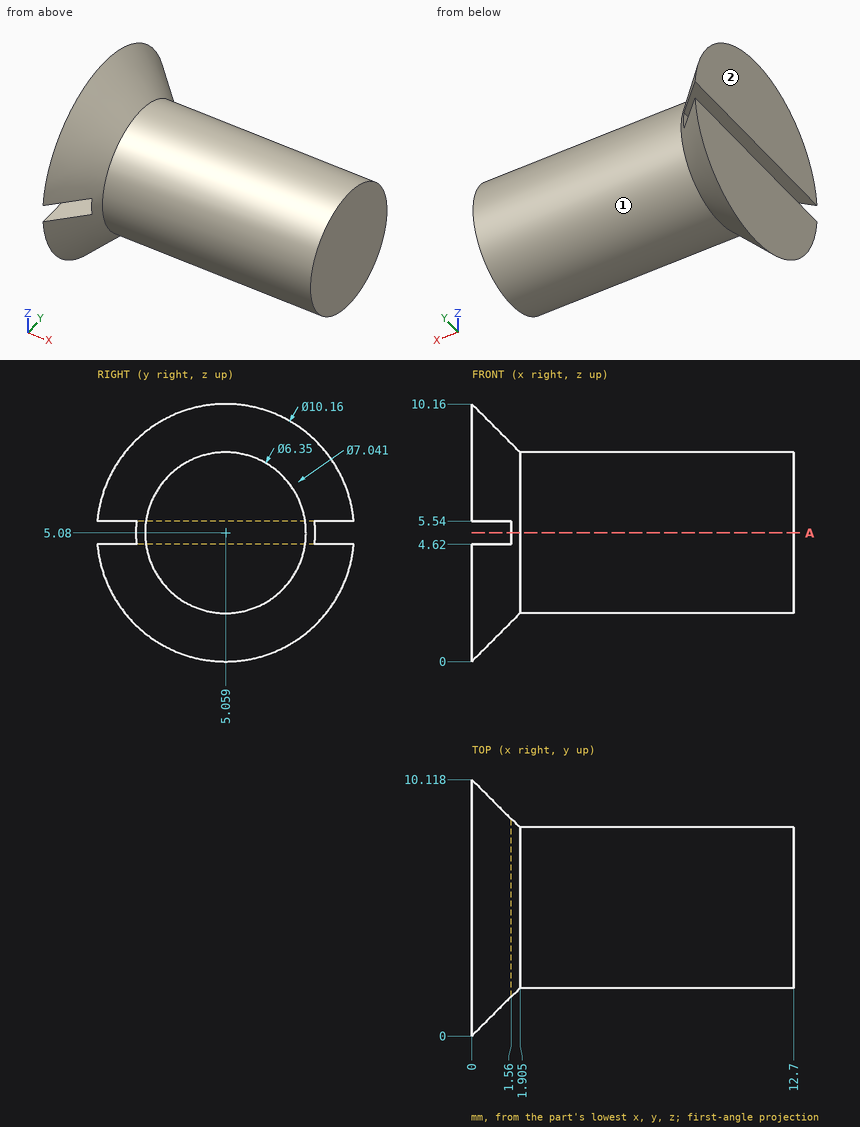
Study the drawing (mm; zero at the part's minimum x, y, z) and answer. A direction names the side the tool comes from. Give positions to 0.01 mm unless a question says otherwise; leave off trailing zeros. Loops run counter-clockwise (first coordinate to the right, second up) from the corner with the lowest first, then second, coordinate; pieces in that order, holes last. Notation, with made-up numbers: (54.5, 46.25) -> (87.5, 46.25) arc R23 cw to (87.5, 75.25) -> close; hole circle Ø2 at (79.5, 49). An arc over 180 degrees is marked (long way). Use a Markdown table: item, result. Add a question column.
1) Which of the six approach directions +Z, -Z, +X, -X, +Y, -Y give full straight-line access (tool end or side, diameter ignored) to the marked faces 1 and 2?
2) Each of these flat-tipped pins is pushed along its axis until it touches: P1, Ø2, axis at x = 10.5, y = 7, coming from the +Z side; P2, Ø1, axis at x = 1.5, z = 7, coming from the +Y side; P3, Ø0.5, axis at x = 0.5, y = 6.5, coming from the +Z side. Where does it stop, or does it pass through?
3) Consider line 1 along Y through (x, z) = (7, 5) (1 decimal); line 2 along X through (y, z) = (4.5, 5.25); line 3 along Y through (x, z) = (12.25, 4) (1 decimal). Determine where each line is inside the solid, lowest interval first.
4) The part is cut by section A-A, the plane z = 5.08. Determine the outline of the cut face in (x, y) (1 decimal).
Reported:
| question | item | result |
|---|---|---|
| 1 | face 1 | +X |
| 1 | face 2 | +Z, -Z, -X, +Y, -Y |
| 2 | P1 | stops at z = 8.11 |
| 2 | P2 | stops at y = 8.71 |
| 2 | P3 | stops at z = 9.7 |
| 3 | line 1 | y = 1.9 to 8.2 |
| 3 | line 2 | x = 1.56 to 12.7 |
| 3 | line 3 | y = 2.1 to 8 |
| 4 | outline | (1.6, 1.5) -> (1.9, 1.9) -> (12.7, 1.9) -> (12.7, 8.2) -> (1.9, 8.2) -> (1.6, 8.6) -> close |
